Verification items for this drawing (mm, ordinates from the low corner). Give positions to 0.01 mm unless a question says otherwise; leave off trailing zeros. Write each loop counter-clockwise with the first axis right and the second up, starting at its lowest first coordinate (ties: lowest second). Pieces come first, ordered by that corner, then holes. Notation, with made-up numbers: M -31,8.5 L -5,8.5 A21 ccw -5,24.5 Z; hole C -14.5,32.25 d5. An arc over 180 degrees is marked long. Write each question's results on one line, items separated by ' | '.
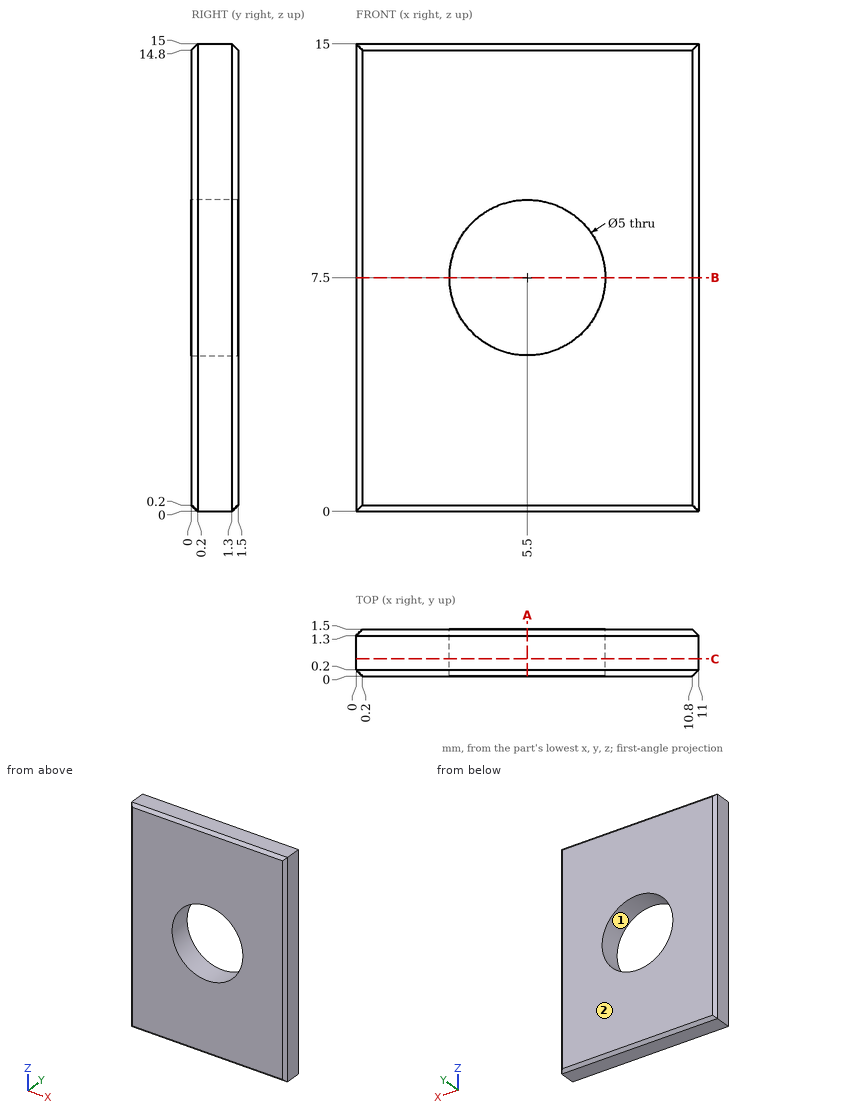
Q1. Material ranges on probe 1 along X at (y, z) = (0.55, 7.5); probe 2 along Z at (x, y) = (4, 0.75); probe 3 along Z at (x, y) = (5.75, 0.5), recorded low to high. Write a range as [from, to].
Answer key:
probe 1: x = [0, 3], [8, 11] | probe 2: z = [0, 5.5], [9.5, 15] | probe 3: z = [0, 5.01], [9.99, 15]
Q2. Depth check by flat-ended pin: P1, Ø6, axis at x = 6.5, z = 9, coming from the +Y side. Enter the tip coordinate at first touch or a pass-through.
Answer key:
P1: stops at y = 1.5
Q3. Section check A-A (x = 5.5). Enter the section's corners in (y, z).
Answer key:
outline: M 0,0.2 L 0.2,0 L 1.3,0 L 1.5,0.2 L 1.5,5 L 0,5 Z; M 0,10 L 1.5,10 L 1.5,14.8 L 1.3,15 L 0.2,15 L 0,14.8 Z
Q4. Section check C-C (y = 0.55). Enter the section's corners in (x, z).
Answer key:
outline: M 0,0 L 11,0 L 11,15 L 0,15 Z; hole C 5.5,7.5 d5
Q5. Section check B-B (z = 7.5). Enter the section's corners in (x, y), then the cut area to 3 significant figures.
Answer key:
outline: M 0,0.2 L 0.2,0 L 3,0 L 3,1.5 L 0.2,1.5 L 0,1.3 Z; M 8,0 L 10.8,0 L 11,0.2 L 11,1.3 L 10.8,1.5 L 8,1.5 Z | area: 8.92 mm2
Q6. Release check for a two-part mould opening along X. For the marked faces 1 and 2 record: released by +X, released by -X, zero draft, split by the parting line, or undercut.
Answer key:
face 1: undercut | face 2: zero draft
